```python
from build123d import *

# Parameters (mm, degrees)
F0_W     = 22
F0_H     = 12
F1_DEPTH = 1
F2_DEPTH = 10
F3_W     = 2.4
F3_H     = 2.5
F4_DEPTH = 9
F5_R     = 2


with BuildPart() as f1:
    # F0 (on Top) → F1 (new body)
    with BuildSketch(Plane.XY):
        Rectangle(F0_W, F0_H)
        Polygon((-5.85, 3.015924), (0, 3.015924), (5.85, 3.015924), (5.85, 0.515924), (8.6, 0.515924), (8.6, -2.484076), (0, -2.484076), (-8.6, -2.484076), (-8.6, 0.515924), (-5.85, 0.515924), align=None, mode=Mode.SUBTRACT)
        Polygon((8.6, 0.515924), (5.85, 0.515924), (-5.85, 0.515924), (-8.6, 0.515924), (-8.6, -2.484076), (0, -2.484076), (8.6, -2.484076), align=None)
    extrude(amount=F1_DEPTH)

    # F0 (on Top) → F2 (join)
    with BuildSketch(Plane.XY):
        Rectangle(F0_W, F0_H)
        Polygon((-5.85, 3.015924), (0, 3.015924), (5.85, 3.015924), (5.85, 0.515924), (8.6, 0.515924), (8.6, -2.484076), (0, -2.484076), (-8.6, -2.484076), (-8.6, 0.515924), (-5.85, 0.515924), align=None, mode=Mode.SUBTRACT)
    extrude(amount=F2_DEPTH)

    # F3 (on face) → F4 (cut, through all)
    with BuildSketch(Plane.XY.offset(10)):
        with Locations((-7.05, 1.765924)):
            Rectangle(F3_W, F3_H)
        with Locations((7.05, 1.765924)):
            Rectangle(F3_W, F3_H)
    extrude(amount=-F4_DEPTH, mode=Mode.SUBTRACT)

    # F5
    f5_edges = [f1.edges().sort_by_distance(p)[0] for p in [
        (-11, -6, 5),
        (11, -6, 5),
        (-11, 6, 5),
        (11, 6, 5),
    ]]
    fillet(f5_edges, radius=F5_R)


solid = f1.part
```
The model under review builds one solid part; all positions refer to its coordinate system, in mm. A direction names the side the tool comes from. Give positions to 0.01 mm unless a question says otherwise; leave off trailing zeros. Write each loop counter-clockwise with the first axis right and the second up, starting at its lowest first coordinate (ties: lowest second). Pieces come first, ordered by that corner, then holes. Notation, with made-up numbers: M -3,35.25 L 49,35.25 A19 ccw 49,57.25 Z; hole C -35,50 d10. An arc over 180 degrees is marked long. Write item = value, one per line. Start each with the question number.
Q1. Machinability: for faces 5 (the face through (-5.85, 1.7, 0.5)), 6 (the face through (11, 0, 5)), 7 (the face through (-8.6, -1, 5)), which of the approach directions +Z, -Z, +X, -X, +Y, -Y give a long, thin tool a straight path to every point of the face, cutting with its end or side? Answer none if there is none.
Q2. For line 1 (X direction, y = 0.75, z = 3.25); line 2 (Y direction, x = -6.5, z = 4); line 3 (Y direction, x = -3, z = 0.75), list the stretches that pass through material, from the lowest coordinate up.
Q3. We need section B-B (z = 3.5). State the section outline as (x, y) points.
Q4. Mouldability with a two-part tool opening along X and no side actions: class faces 1 (the face through (10.43, -5.4, 5.07)), 2 (the face through (-10.43, -5.4, 5.07)), 3 (the face through (0.1, 0.516, 0.5)), 4 (the face through (-8.25, 2, 6)) as released by +X, released by -X, zero draft, split by the parting line, or undercut.
Q5. We need section C-C (y = 0.75). State the section outline as (x, z) points.
Q6. Clearance check with a flat-ended pin moving along its axis: pin 1 (3 mm diameter, centred on x = 0.5, y = 1, fed in from +Z). State where the tip first meets the part, or that it passes through.
Q7. We need section A-A (x = -1.75). State the section outline as (y, z) points, plus the area to 3 significant figures.
Q8. We need section D-D (y = 5.25). State the section outline as (x, z) points.
Result set:
q1.face_5 = +Z, -Z
q1.face_6 = +Z, -Z, +X, +Y, -Y
q1.face_7 = +Z
q2.line_1 = -11 to -8.25, 8.25 to 11
q2.line_2 = -6 to -2.48, 3.02 to 6
q2.line_3 = -6 to 0.52, 3.02 to 6
q3.outline = M -11,-4 A2 ccw -9,-6 L 9,-6 A2 ccw 11,-4 L 11,4 A2 ccw 9,6 L -9,6 A2 ccw -11,4 Z; hole M -8.6,-2.48 L 8.6,-2.48 L 8.6,0.52 L 8.25,0.52 L 8.25,3.02 L -8.25,3.02 L -8.25,0.52 L -8.6,0.52 Z
q4.face_1 = released by +X
q4.face_2 = released by -X
q4.face_3 = undercut
q4.face_4 = undercut
q5.outline = M -11,0 L -5.85,0 L -5.85,1 L -8.25,1 L -8.25,10 L -11,10 Z; M 5.85,0 L 11,0 L 11,10 L 8.25,10 L 8.25,1 L 5.85,1 Z
q6.pin_1 = 1
q7.outline = M -6,0 L 0.52,0 L 0.52,1 L -2.48,1 L -2.48,10 L -6,10 Z; M 3.02,0 L 6,0 L 6,10 L 3.02,10 Z
q7.area = 68.0 mm2
q8.outline = M -10.56,0 L 10.56,0 L 10.56,10 L -10.56,10 Z
